Autodesk Inventor part; units mm, degrees
ref_plane "YZ Plane" through (0, 0, 0) normal (1, 0, 0) x (0, 1, 0)
ref_plane "XZ Plane" through (0, 0, 0) normal (0, 1, 0) x (-1, 0, 0)
ref_plane "XY Plane" through (0, 0, 0) normal (0, 0, 1) x (1, 0, 0)
sketch "Sketch1" plane through (0, 0, 0) normal (0, 0, 1) x (1, 0, 0)
  circle A0 centre (4, 9.5) radius 1.75
  circle A1 centre (4, 4) radius 1.75
  line L0 (4, 9.5) -> (4, 4) construction
  line L1 (0.75, 6.75) -> (0.75, 13.5)
  line L2 (0.75, 13.5) -> (7.25, 13.5)
  line L3 (7.25, 13.5) -> (7.25, 6.75)
  line L4 (0, 6.75) -> (0, 0)
  line L5 (0, 0) -> (8, 0)
  line L6 (8, 0) -> (8, 6.75)
  line L7 (0, 6.75) -> (0.75, 6.75)
  line L8 (7.25, 6.75) -> (8, 6.75)
  line L9 (0.75, 6.75) -> (7.25, 6.75) construction
  line L10 (4, 4) -> (4, 0) construction
  line L11 (4, 9.5) -> (4, 13.5) construction
  point P0 (4, 6.75)
  dimension "d0" = 3.5
  dimension "d1" = 3.5
  dimension "d2" = 5.5
  dimension "d3" = 6.5
  dimension "d4" = 8
  dimension "d5" = 13.5
extrude "Extrusion1" add sketch "Sketch1" along normal blind 7
fillet "Fillet1" radius 0.8 8 edges at (7.25, 13.5, 3.5) (0.75, 13.5, 3.5) (8, 0, 3.5) (0, 0, 3.5) (0.75, 6.75, 3.5) (0, 6.75, 3.5) (8, 6.75, 3.5) (7.25, 6.75, 3.5)
properties part number "Tplug"
Verification items for the finished model (mm, model axes). A direction names the side the tool comes from. Coordinates: 2 decimals unless noted, no trailing zeros. Loops run counter-clockwise (first coordinate to the right, second up) from the corner with the lowest first, then second, coordinate; pieces in that order, holes last. Notation, with made-up numbers: (70, 66.5) -> (126, 66.5) arc R34 cw to (126, 98.5) -> close; hole circle Ø7 at (68, 76). An arc over 180 degrees is marked (long way). Write each question's results on one line, items separated by ' | '.
Item 1: Section check A-A, the plane x = 4. Enter the section's corners in (y, z), plus the area to 3 significant figures.
Found:
outline: (0, 0) -> (2.25, 0) -> (2.25, 7) -> (0, 7) -> close; (5.75, 0) -> (7.75, 0) -> (7.75, 7) -> (5.75, 7) -> close; (11.25, 0) -> (13.5, 0) -> (13.5, 7) -> (11.25, 7) -> close | area: 45.5 mm2
Item 2: Tool access check on faces 5 (the face through (8, 3, 3)), 6 (the face through (0.75, 10, 3)). Record the directions out of +Z, -Z, +X, -X, +Y, -Y that give a thin tool (end or side, any length) a straight path to the whole face; none if there is none.
Found:
face 5: +Z, -Z, +X, +Y, -Y | face 6: +Z, -Z, -X, +Y
Item 3: Section check C-C, the plane y = 9.5. Enter the section's corners in (x, z), plus the area to 3 significant figures.
Found:
outline: (0.75, 0) -> (2.25, 0) -> (2.25, 7) -> (0.75, 7) -> close; (5.75, 0) -> (7.25, 0) -> (7.25, 7) -> (5.75, 7) -> close | area: 21.0 mm2
Item 4: Gauge pin test, flat ends, axial feed: pin 1 (1 mm diameter, centred on x = 5, y = 8, fed in from -Z); pin 2 (4 mm diameter, centred on y = 10.5, z = 3, fed in from +X); pin 3 (3 mm diameter, centred on x = 4, y = 4, fed in from -Z); pin 4 (1.5 mm diameter, centred on y = 11, z = 4.5, fed in from -X). Record the tip position at first contact, or that the pin passes through.
Found:
pin 1: stops at z = 0 | pin 2: stops at x = 7.25 | pin 3: passes through | pin 4: stops at x = 0.75
Item 5: Section check B-B, the plane z = 3.25. Enter the section's corners in (x, y) (3 decimals), plus the area to 3 significant figures.
Found:
outline: (0, 0.8) arc R0.8 ccw to (0.8, 0) -> (7.2, 0) arc R0.8 ccw to (8, 0.8) -> (8, 6.193) arc R0.8 ccw to (7.625, 6.871) arc R0.8 cw to (7.25, 7.548) -> (7.25, 12.7) arc R0.8 ccw to (6.45, 13.5) -> (1.55, 13.5) arc R0.8 ccw to (0.75, 12.7) -> (0.75, 7.548) arc R0.8 cw to (0.375, 6.871) arc R0.8 ccw to (0, 6.193) -> close; hole circle Ø3.5 at (4, 4); hole circle Ø3.5 at (4, 9.5) | area: 78.3 mm2
Item 6: Section check D-D, the plane y = 4. Enter the section's corners in (x, z), plus the area to 3 significant figures.
Found:
outline: (0, 0) -> (2.25, 0) -> (2.25, 7) -> (0, 7) -> close; (5.75, 0) -> (8, 0) -> (8, 7) -> (5.75, 7) -> close | area: 31.5 mm2
Item 7: Mould release check, pull along X, two halves, no side actions. Record for faces 1 (the face through (2.25, 3.92, 3.45)), 2 (the face through (7.25, 10, 3)), 3 (the face through (4, 7, 7)), 4 (the face through (2.71, 8.32, 3.45)): +X half, -X half, draft (parallel to the pull), parting line (faces both ways), or undercut.
Found:
face 1: undercut | face 2: +X half | face 3: draft | face 4: undercut
Item 8: Material ranges on L1, parallel to Y at x = 4, z = 5; L2, parallel to Y at x = 2.75, z = 6.5; L3, parallel to X at y = 10.5, z = 1.5, recorded low to high.
Found:
L1: y = 0 to 2.25, 5.75 to 7.75, 11.25 to 13.5 | L2: y = 0 to 2.78, 5.22 to 8.28, 10.72 to 13.5 | L3: x = 0.75 to 2.56, 5.44 to 7.25
